Geometry: see drawing. Coordinates: mm, zero at the bounding-box minimum. Give positions to 0.01 mm unless a question says otherwise; leave off trailing zeros. Order: outer loops, then holes, each group sorted by start corner. A loop starts at its lowest first (then second) coordinate and runs counter-clockwise, first axis right, second up. Notation, with made-up numbers: (-18.5, -39) - (7.5, -39) arc R25 cw to (7.5, -22) - close; hole circle Ø2 at (-22.75, -3). An arc over 180 degrees is marked (long way). One line per question, with ' | ' between items. Start each with the question number.
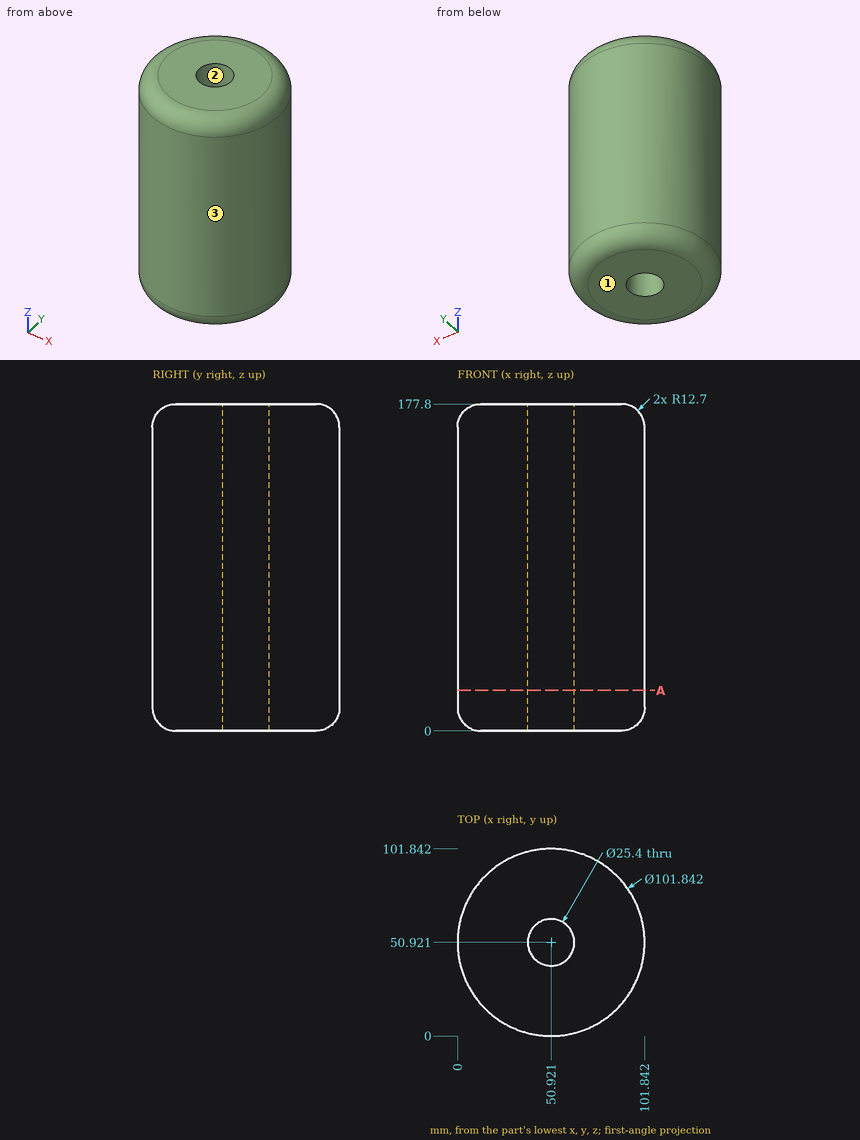
(1) Pull-direction query (Y, two-part tool) for the marked faces 1, 2 and 3; classes: +Y half, -Y half, draft (parallel to the pull), parting line (faces both ways), or undercut.
(2) Material intervals for line 1 along Y through (x, z) = (50, 149.5); line 2 along X through (y, z) = (57, 9); line 3 along Y through (x, z) = (68, 101), sorted ascending. Write a range as from..to.
(3) Contact query for flat-ended pins moving along their axis: P1, Ø12, axis at x = 13, z = 147, coming from the -Y side; P2, Ø2, axis at y = 88.5, z = 149, coming from the -X side; P3, Ø2, axis at x = 78, y = 10.5, coming from the -Z side. Output: stop coordinate, or through.
(4) Cut plane A-A, the plane z = 22. Return the cut outline in (x, y), plus the area to 3 significant figures.
Results are:
1) face 1: draft | face 2: undercut | face 3: parting line
2) line 1: 0.01..38.25, 63.59..101.83 | line 2: 0.92..39.77, 62.07..100.92 | line 3: 2.95..98.89
3) P1: y = 11.25 | P2: x = 15.5 | P3: z = 4.2
4) outline: circle Ø101.84 at (50.92, 50.92); hole circle Ø25.4 at (50.92, 50.92) | area: 7,640 mm2
